Autodesk Inventor part; units mm, degrees
ref_plane "YZ Plane" through (0, 0, 0) normal (1, 0, 0) x (0, 1, 0)
ref_plane "XZ Plane" through (0, 0, 0) normal (0, 1, 0) x (-1, 0, 0)
ref_plane "XY Plane" through (0, 0, 0) normal (0, 0, 1) x (1, 0, 0)
sketch "Sketch1" plane through (0, 0, 0) normal (0, 0, 1) x (1, 0, 0)
  line L0 (-12.245, 11.65) -> (-12.245, 3)
  line L1 (-12.245, 3) -> (-45.245, 3)
  line L2 (-45.245, 3) -> (-45.245, 0)
  line L3 (-45.245, 0) -> (-10.245, 0)
  line L4 (-10.245, 0) -> (-10.245, 8.8)
  line L5 (-10.245, 8.8) -> (10.245, 8.8)
  line L6 (10.245, 8.8) -> (10.245, 0)
  line L7 (10.245, 0) -> (45.245, 0)
  line L8 (45.245, 0) -> (45.245, 3)
  line L9 (45.245, 3) -> (12.245, 3)
  line L10 (12.245, 3) -> (12.245, 11.65)
  line L11 (12.245, 11.65) -> (-12.245, 11.65)
  line L12 (-10.245, 0) -> (10.245, 0) construction
  point P0 (0, 0)
  point P1 (0, 11.65)
  point P2 (0, 0)
  point P3 (-12.245, 7.325)
  point P4 (12.245, 7.325)
  dimension "d0" = 20.49
  dimension "d1" = 2.85
  dimension "d3" = 5.8
  dimension "d4" = 3
  dimension "d5" = 3
  dimension "d6" = 35
  dimension "d7" = 35
  dimension "d73" = 33
  dimension "d74" = 33
extrude "Extrusion1" add sketch "Sketch1" along normal mid plane 41.1
sketch "Sketch8" plane through (12.245, 3, 20.55) normal (0, 1, 0) x (1, 0, 0)
  line L0 (0, 41.1) -> (0, 0)
  line L1 (33, 0) -> (0, 0)
  line L2 (33, 41.1) -> (33, 0)
  line L3 (0, 41.1) -> (33, 41.1)
  line L4 (-57.49, 41.1) -> (-57.49, 0)
  line L5 (-24.49, 0) -> (-57.49, 0)
  line L6 (-24.49, 0) -> (-24.49, 41.1)
  line L7 (-57.49, 41.1) -> (-24.49, 41.1)
  line L8 (33, 41.1) -> (33, 0)
  circle A0 centre (-11.645, 30.6) radius 6.4
  line L9 (-12.245, 41) -> (-12.245, 0) construction
  point P0 (-12.245, 20.55)
  point P1 (-54.49, 30.65)
  point P2 (-29.49, 30.65)
  point P3 (-57.49, 20.55)
  point P4 (30, 30.65)
  point P5 (5, 30.65)
  dimension "d42" = 3
  dimension "d43" = 25
  dimension "d51" = 10.45
  dimension "d53" = 3
hole "Hole1" at (-42.245, 3, -10.1) at (-17.245, 3, -10.1) at (17.245, 3, -10.1) at (42.245, 3, -10.1) direction (0, -1, 0) diameter 2.459 end through all
sketch "Sketch9" plane through (12.245, 3, 20.55) normal (0, 1, 0) x (1, 0, 0)
  circle A0 centre (30, 30.65) radius 1.2295
  circle A1 centre (5, 30.65) radius 1.2295
  line L0 (0, 41.1) -> (0, 0)
  line L1 (33, 0) -> (0, 0)
  line L2 (33, 41.1) -> (33, 0)
  line L3 (0, 41.1) -> (33, 41.1)
  arc A2 (33, 24) -> (9, 0) centre (33, 0) ccw
  point P0 (-12.245, 20.55)
  dimension "d60" = 24
extrude "Extrusion2" cut sketch "Sketch9" against normal blind 10 contours A2 L2 L1
mirror "Mirror1" about plane through (0, 0, 0) normal (1, 0, 0) of "Extrusion2"
sketch "Sketch10" plane through (-12.245, 11.65, 20.55) normal (0, 1, 0) x (1, 0, 0)
  circle A0 centre (12.245, 30.602) radius 6.5
  line L0 (0, 41.1) -> (0, 0)
  line L1 (24.49, 0) -> (0, 0)
  line L2 (24.49, 41.1) -> (24.49, 0)
  line L3 (0, 41.1) -> (24.49, 41.1)
  point P0 (12.245, 20.55)
  point P1 (12.245, 41.1)
  dimension "d75" = 13
  dimension "d76" = 10.498
extrude "Extrusion3" cut sketch "Sketch10" against normal blind 10 contours A0
sketch "Sketch11" plane through (-12.245, 11.65, 20.55) normal (0, 1, 0) x (1, 0, 0)
  circle A0 centre (5.245, 10.482) radius 0.7835
  circle A1 centre (4.245, 23.702) radius 0.7835
  circle A2 centre (4.175, 38.602) radius 0.7835
  circle A3 centre (20.315, 38.602) radius 0.7835
  circle A4 centre (20.245, 23.702) radius 0.7835
  circle A5 centre (19.245, 10.482) radius 0.7835
hole "Hole2" at (-8, 11.65, -3.152) at (8, 11.65, -3.152) at (8.07, 11.65, -18.052) at (-8.07, 11.65, -18.052) at (-7, 11.65, 10.068) at (7, 11.65, 10.068) direction (0, -1, 0) diameter 2.1 end through all counterbore diameter 4.1 counterbore depth 1.4
fillet "Fillet3" radius 3 6 edges at (-21.245, 1.5, 20.55) (-45.245, 1.5, -3.45) (-45.245, 1.5, -20.55) (21.245, 1.5, 20.55) (45.245, 1.5, -3.45) (45.245, 1.5, -20.55)
ref_plane "Work Plane1" through (0, 0, 0) normal (1, 0, 0) x (0, 1, 0)
properties part number "gripper_fixer" material "Aluminum 6061-AHC"
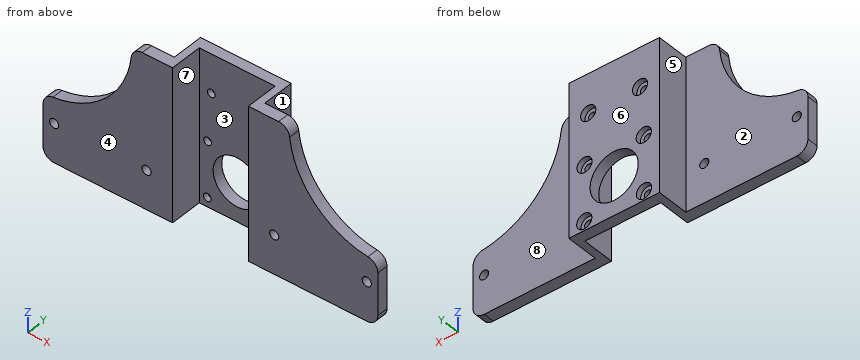
Can you work these out from the model? Positions are in its coordinate system, mm. Face numbers are marked on the shaded views. A direction names the side the tool comes from. Coordinates: 2 decimals unless noted, no trailing zeros. Write each loop counter-clockwise with the first axis right and the second up, starting at its lowest first coordinate (ties: lowest second). Pieces come first, ordered by that corner, then holes. Notation, with made-up numbers: M -3.5,24 L 36.5,24 A28 ccw 36.5,61 Z; hole C 88,70 d3. An arc over 180 degrees is marked long. Answer as CSV lines item,"result".
Item 1: Please list where these lines run through material, in increasing order: line 1 along X through (y, z) = (7.5, 6) (3 decimals); line 2 along Z through (x, y) = (0, 9.5); line 3 along X through (y, z) = (1.55, -10.1) (1 decimal).
Geometry results:
line 1,"x = -12.245 to -10.245, 10.245 to 12.245"
line 2,"z = -20.55 to -16.55, -3.55 to 20.55"
line 3,"x = -45.2 to -43.5, -41 to -18.5, -16 to -10.2, 10.2 to 16, 18.5 to 41, 43.5 to 45.2"
Item 2: Imagine slicing it at A-A on x = 0. List the corners of the cut face in (y, z) for me, plus the area to 3 significant figures.
Geometry results:
outline,"M 8.8,-20.55 L 11.65,-20.55 L 11.65,-16.55 L 8.8,-16.55 Z; M 8.8,-3.55 L 11.65,-3.55 L 11.65,20.55 L 8.8,20.55 Z"
area,"80.1 mm2"
Item 3: Imagine slicing it at D-D on z = 4. List the corners of the cut face in (x, y) for me (3 decimals), plus the area to 3 significant figures.
Geometry results:
outline,"M -27.864,0 L -10.245,0 L -10.245,8.8 L 10.245,8.8 L 10.245,0 L 27.864,0 L 27.864,3 L 12.245,3 L 12.245,11.65 L -12.245,11.65 L -12.245,3 L -27.864,3 Z"
area,"199 mm2"
Item 4: I'm going to push flat-ended pins straight in: P1, Ø1.5, axis at x = -26, y = 4, coming from the -Z side; P2, Ø4, axis at x = 42.245, z = -10.1, coming from the +Y side; P3, Ø3.5, axis at x = -8.07, z = -18.052, coming from the -Y side; P4, Ø2.5, axis at x = 7, z = 10.068, coming from the +Y side. Where does each tip first touch, or does it pass through?
Geometry results:
P1,"passes through"
P2,"stops at y = 3"
P3,"stops at y = 8.8"
P4,"stops at y = 10.25"
Item 5: Imagine slicing it at B-B on y = 4.25. List the corners of the cut face in (x, z) for me (3 decimals).
Geometry results:
outline,"M -12.245,-20.55 L -10.245,-20.55 L -10.245,20.55 L -12.245,20.55 Z; M 10.245,-20.55 L 12.245,-20.55 L 12.245,20.55 L 10.245,20.55 Z"
Item 6: We'd pull the mould along X, two halves only. Please class the marked faces 1, 2 and 3: +X half, -X half, draft (parallel to the pull), parting line (faces both ways), or undercut.
Geometry results:
face 1,"+X half"
face 2,"draft"
face 3,"undercut"
Item 7: On a 3-axis mill with a long thin cutter (end or side, diameter ignored), from which of +Z, -Z, +X, -X, +Y, -Y can I reach the whole of each face in a straight line? I mean the marked faces 4, 5, 6, 7 and 8. Say none if no direction works.
Geometry results:
face 4,"+Z, -Z, +X, -X, -Y"
face 5,"+Z, -Z, -X, +Y"
face 6,"+Z, -Z, +X, -X, +Y"
face 7,"+Z, -Z, -Y"
face 8,"+Z, -Z, +X, +Y"
Item 8: Imagine slicing it at C-C on z = -14. List the corners of the cut face in (x, y) for me (3 decimals).
Geometry results:
outline,"M -45.245,0 L -10.245,0 L -10.245,8.8 L -5.164,8.8 L -5.164,11.65 L -12.245,11.65 L -12.245,3 L -45.245,3 Z; M 5.164,8.8 L 10.245,8.8 L 10.245,0 L 45.245,0 L 45.245,3 L 12.245,3 L 12.245,11.65 L 5.164,11.65 Z"
